from build123d import *

# Parameters (mm, degrees)
SKETCH_1_W           = 6
SKETCH_1_H           = 56.5
SKETCH_1_R           = 1.25
EXTRUDE_1_DEPTH      = 4
SKETCH_1_H_2         = 41
EXTRUDE_1_2_DEPTH    = 4
SKETCH_3_W           = 3
SKETCH_3_H           = 103.5
EXTRUDE_2_DEPTH      = 33
SKETCH_1_5_R         = 2
CUT_EXTRUDE_1_DEPTH  = 1.5
EXTRUDE_3_REACH      = 90.366
SKETCH_4_W           = 82.8
SKETCH_4_H           = 3
SKETCH_5_W           = 76.8
SKETCH_5_H           = 3
CUT_EXTRUDE_2_DEPTH  = 3.2
SKETCH_7_W           = 79.8
SKETCH_7_H           = 1.2
CUT_EXTRUDE_4_DEPTH  = 113.495377683
SKETCH_8_R           = 0.9
CUT_EXTRUDE_5_DEPTH  = 89.365844646
SKETCH_9_R           = 0.6
CUT_EXTRUDE_6_DEPTH  = 116.183375537
SKETCH_9_3_R         = 1
CUT_EXTRUDE_7_DEPTH  = 1.5
SKETCH_10_R          = 0.35
CUT_EXTRUDE_8_DEPTH  = 3
SKETCH_11_R          = 0.35
CUT_EXTRUDE_9_DEPTH  = 3
SKETCH_12_R          = 0.35
CUT_EXTRUDE_10_DEPTH = 116.183375537


with BuildPart() as part:
    # Sketch 1 → Extrude 1 (new body)
    with BuildSketch(Plane(origin=(0, 0, 0), x_dir=(1, 0, 0), z_dir=(0, 1, 0))):
        with Locations((-35.4, -4.5)):
            Rectangle(SKETCH_1_W, SKETCH_1_H)
        with Locations(Location((-35.4, 20.75, 0), (0, 0, 270))):
            Circle(SKETCH_1_R, mode=Mode.SUBTRACT)
        with Locations(Location((-35.4, -20.75, 0), (0, 0, 270))):
            Circle(SKETCH_1_R, mode=Mode.SUBTRACT)
    extrude(amount=EXTRUDE_1_DEPTH)



with BuildPart() as body_2:
    # Sketch 1 → Extrude 1 2 (new body)
    with BuildSketch(Plane(origin=(0, 0, 0), x_dir=(1, 0, 0), z_dir=(0, 1, 0))):
        with Locations((-35.4, 50.25)):
            Rectangle(SKETCH_1_W, SKETCH_1_H_2)
    extrude(amount=EXTRUDE_1_2_DEPTH)


with BuildPart() as part_1:
    add(part.part)

    add(body_2.part)  # Extrude 2 merges body 2
    # Sketch 3 → Extrude 2 (add)
    with BuildSketch(Plane(origin=(0, 4, 0), x_dir=(1, 0, 0), z_dir=(0, 1, 0))):
        with Locations((-39.9, 19)):
            Rectangle(SKETCH_3_W, SKETCH_3_H)
    extrude(amount=-EXTRUDE_2_DEPTH)

    # Sketch 1_5 → Cut-Extrude 1 (cut)
    with BuildSketch(Plane(origin=(0, 0, 0), x_dir=(1, 0, 0), z_dir=(0, 1, 0))):
        with Locations(Location((-35.4, 20.75, 0), (0, 0, 270))):
            Circle(SKETCH_1_5_R)
        with Locations(Location((-35.4, -20.75, 0), (0, 0, 270))):
            Circle(SKETCH_1_5_R)
    extrude(amount=CUT_EXTRUDE_1_DEPTH, mode=Mode.SUBTRACT)


with BuildPart() as body_2_2:
    # Mirror 3: mirrored copy
    add(part_1.part.mirror(Plane(origin=(0, 0, 0), x_dir=(0, 0, 1), z_dir=(1, 0, 0))))

    # Extrude 3: up to this face of the body (flat: up to its plane)
    extrude_3_end = Plane(body_2_2.part.faces().sort_by_distance((39.9, -29, -19))[0])
    # Sketch 4 → Extrude 3 (add, up to the picked face)
    with BuildSketch(Plane.XZ.offset(-4), mode=Mode.PRIVATE) as extrude_3_sk1:
        with Locations((0, 31.25)):
            Rectangle(SKETCH_4_W, SKETCH_4_H)
    extrude_3_tool1 = split(extrude(extrude_3_sk1.sketch, amount=EXTRUDE_3_REACH, mode=Mode.PRIVATE), bisect_by=extrude_3_end, keep=Keep.BOTH, mode=Mode.PRIVATE)
    # Sketch 4 → Extrude 3 (add, up to the picked face)
    with BuildSketch(Plane.XZ.offset(-4), mode=Mode.PRIVATE) as extrude_3_sk2:
        with Locations((0, -69.25)):
            Rectangle(SKETCH_4_W, SKETCH_4_H)
    extrude_3_tool2 = split(extrude(extrude_3_sk2.sketch, amount=EXTRUDE_3_REACH, mode=Mode.PRIVATE), bisect_by=extrude_3_end, keep=Keep.BOTH, mode=Mode.PRIVATE)

    add(part_1.part)  # Extrude 3 merges part
    add(extrude_3_tool1.solids().sort_by(Axis((0, 4, 31.25), (0, -1, 0)))[0])
    add(extrude_3_tool2.solids().sort_by(Axis((0, 4, -69.25), (0, -1, 0)))[0])

    # Sketch 5 → Cut-Extrude 2 (cut)
    with BuildSketch(Plane.XZ.offset(29)):
        with Locations((0, 31.25)):
            Rectangle(SKETCH_5_W, SKETCH_5_H)
    extrude(amount=-CUT_EXTRUDE_2_DEPTH, mode=Mode.SUBTRACT)

    # Sketch 7 → Cut-Extrude 4 (cut, through all)
    with BuildSketch(Plane.XY.offset(-67.75)):
        with Locations((0, -26.4)):
            Rectangle(SKETCH_7_W, SKETCH_7_H)
    extrude(amount=CUT_EXTRUDE_4_DEPTH, mode=Mode.SUBTRACT)

    # Sketch 8 → Cut-Extrude 5 (cut, through all)
    with BuildSketch(Plane(origin=(0, 4, 0), x_dir=(1, 0, 0), z_dir=(0, 1, 0))):
        with Locations(Location((36.9, 62.75, 0), (0, 0, 270))):
            Circle(SKETCH_8_R)
        with Locations(Location((-36.9, 62.75, 0), (0, 0, 270))):
            Circle(SKETCH_8_R)
        with Locations(Location((-36.9, 42.75, 0), (0, 0, 270))):
            Circle(SKETCH_8_R)
        with Locations(Location((36.9, 42.75, 0), (0, 0, 270))):
            Circle(SKETCH_8_R)
    extrude(amount=-CUT_EXTRUDE_5_DEPTH, mode=Mode.SUBTRACT)

    # Sketch 9 → Cut-Extrude 6 (cut, through all)
    with BuildSketch(Plane(origin=(0, 0, -70.75), x_dir=(-1, 0, 0), z_dir=(0, 0, -1))):
        with Locations((13.8, -27.5)):
            Circle(SKETCH_9_R)
        with Locations((-13.8, -27.5)):
            Circle(SKETCH_9_R)
    extrude(amount=-CUT_EXTRUDE_6_DEPTH, mode=Mode.SUBTRACT)

    # Sketch 9_3 → Cut-Extrude 7 (cut)
    with BuildSketch(Plane(origin=(0, 0, -70.75), x_dir=(-1, 0, 0), z_dir=(0, 0, -1))):
        with Locations((-13.8, -27.5)):
            Circle(SKETCH_9_3_R)
        with Locations((13.8, -27.5)):
            Circle(SKETCH_9_3_R)
    extrude(amount=-CUT_EXTRUDE_7_DEPTH, mode=Mode.SUBTRACT)

    # Sketch 10 → Cut-Extrude 8 (cut)
    with BuildSketch(Plane.XZ.offset(25.8)):
        with Locations(Location((-13.8, 31.25, 0), (0, 0, 270))):
            Circle(SKETCH_10_R)
        with Locations(Location((13.8, 31.25, 0), (0, 0, 270))):
            Circle(SKETCH_10_R)
    extrude(amount=-CUT_EXTRUDE_8_DEPTH, mode=Mode.SUBTRACT)

    # Sketch 11 → Cut-Extrude 9 (cut)
    with BuildSketch(Plane.XZ.offset(29)):
        with Locations(Location((39.9, 12.05, 0), (0, 0, 270))):
            Circle(SKETCH_11_R)
        with Locations(Location((39.9, -8.65, 0), (0, 0, 270))):
            Circle(SKETCH_11_R)
        with Locations(Location((39.9, -29.35, 0), (0, 0, 270))):
            Circle(SKETCH_11_R)
        with Locations(Location((39.9, -50.05, 0), (0, 0, 270))):
            Circle(SKETCH_11_R)
        with Locations(Location((-39.9, 12.05, 0), (0, 0, 270))):
            Circle(SKETCH_11_R)
        with Locations(Location((-39.9, -8.65, 0), (0, 0, 270))):
            Circle(SKETCH_11_R)
        with Locations(Location((-39.9, -29.35, 0), (0, 0, 270))):
            Circle(SKETCH_11_R)
        with Locations(Location((-39.9, -50.05, 0), (0, 0, 270))):
            Circle(SKETCH_11_R)
    extrude(amount=-CUT_EXTRUDE_9_DEPTH, mode=Mode.SUBTRACT)

    # Sketch 12 → Cut-Extrude 10 (cut, through all)
    with BuildSketch(Plane(origin=(0, 0, -70.75), x_dir=(-1, 0, 0), z_dir=(0, 0, -1))):
        with Locations((-24.84, -6)):
            Circle(SKETCH_12_R)
        with Locations((-8.28, -6)):
            Circle(SKETCH_12_R)
        with Locations((8.28, -6)):
            Circle(SKETCH_12_R)
        with Locations((24.84, -6)):
            Circle(SKETCH_12_R)
        with Locations((-24.84, -19)):
            Circle(SKETCH_12_R)
        with Locations((-8.28, -19)):
            Circle(SKETCH_12_R)
        with Locations((8.28, -19)):
            Circle(SKETCH_12_R)
        with Locations((24.84, -19)):
            Circle(SKETCH_12_R)
    extrude(amount=-CUT_EXTRUDE_10_DEPTH, mode=Mode.SUBTRACT)


solid = body_2_2.part
Geometry check sheet. Reference: the model listing, model coordinates, mm. A direction names the side the tool comes from. Coordinates: 2 decimals unless noted, no trailing zeros. Order: outer loops, then holes, each group sorted by start corner. A loop starts at its lowest first (then second) coordinate and runs counter-clockwise, first axis right, second up. Notation, with made-up numbers: (23.25, 4) - (44.25, 4) arc R19 cw to (44.25, 16) - close; hole circle Ø11 at (58.25, -15.75). An arc over 180 degrees is marked (long way). Answer in a Markdown table with one row per item. Add a question column.
1) Cross-section at B-B, the plane z = -0.5. Record the cut outline in (x, y).
2) Gauge pin test, flat ends, axial feed: P1, Ø5, axis at x = -35.5, z = 0.5, coming from the -Y side; P2, Ø4, axis at x = 30, z = -58.5, coming from the -Y side. Record the tip position at first contact, or that the pin passes through.
3) Cross-section at C-C, the plane y = -14.5. Record the cut outline in (x, z).
4) Set-up check for faces 5 (the flat face through (0, -29, -69)), 6 (the flat face through (35, 2, -23.75)), 7 (the flat face through (35, 0, 3)): record each of +Z, -Z, +X, -X, +Y, -Y from which the full face is reachable in a straight line by a thin tool's end or side.
5) Release check for a two-part mould opening along Y. For faces 1 (the flat face through (-35, 0, -49)), 2 (the flat face through (35, 2, -29.75)), 3 (the flat face through (-39, -25.8, 5)), 4 (the flat face through (-34, 4, -15)) record: +Y half, -Y half, draft (parallel to the pull), parting line (faces both ways), or undercut.
6) Cross-section at A-A, the plane x = -30.5. Record the cut outline in (y, z).
7) Material ranges on line 1 along X through (y, z) = (-19, -69); line 2 along Z through (x, y) = (-39.9, -27.5); line 3 along Z through (x, y) = (36.9, 1.55), recorded low to high. Write a range as [from, to].
Check result:
| question | item | result |
|---|---|---|
| 1 | outline | (-41.4, -29) - (-38.4, -29) - (-38.4, -27) - (-39.9, -27) - (-39.9, -25.8) - (-38.4, -25.8) - (-38.4, 0) - (-32.4, 0) - (-32.4, 4) - (-41.4, 4) - close; (32.4, 0) - (38.4, 0) - (38.4, -25.8) - (39.9, -25.8) - (39.9, -27) - (38.4, -27) - (38.4, -29) - (41.4, -29) - (41.4, 4) - (32.4, 4) - close |
| 2 | P1 | stops at y = 0 |
| 2 | P2 | passes through |
| 3 | outline | (-41.4, -70.75) - (41.4, -70.75) - (41.4, 32.75) - (-41.4, 32.75) - close; hole (-38.4, -67.75) - (38.4, -67.75) - (38.4, 29.75) - (-38.4, 29.75) - close |
| 4 | face 5 | +Z, -Z, +X, -X, -Y |
| 4 | face 6 | +Y, -Y |
| 4 | face 7 | -Y |
| 5 | face 1 | -Y half |
| 5 | face 2 | draft |
| 5 | face 3 | undercut |
| 5 | face 4 | +Y half |
| 6 | outline | (-29, -70.75) - (4, -70.75) - (4, -67.75) - (-29, -67.75) - close; (-25.8, 29.75) - (4, 29.75) - (4, 32.75) - (-25.8, 32.75) - close |
| 7 | line 1 | x = [-41.4, -25.19], [-24.49, -8.63], [-7.93, 7.93], [8.63, 24.49], [25.19, 41.4] |
| 7 | line 2 | z = [-70.75, -50.4], [-49.7, -29.7], [-29, -9], [-8.3, 11.7], [12.4, 32.75] |
| 7 | line 3 | z = [-70.75, -63.65], [-61.85, -43.65], [-41.85, -29.75], [-23.75, 32.75] |
